Model file for the job. Use its own axes, mm. A direction names the side the tool comes from. Round coordinates to 2 decimals unless told otherwise and drop trailing zeros. Order: outer loops, then holes, each group sorted by start corner. A loop starts at its lowest first (then second) coordinate and runs counter-clockwise, first axis right, second up. Notation, with made-up numbers: (-8, 12) - (43, 12) arc R23 ccw to (43, 26) - close; hole circle Ø8 at (80, 82). An arc over 180 degrees is marked (long way). Write item = value, one per line.
Autodesk Inventor part; units mm, degrees
ref_plane "YZ Plane" through (0, 0, 0) normal (1, 0, 0) x (0, 1, 0)
ref_plane "XZ Plane" through (0, 0, 0) normal (0, 1, 0) x (-1, 0, 0)
ref_plane "XY Plane" through (0, 0, 0) normal (0, 0, 1) x (1, 0, 0)
sketch "草圖1" plane through (0, 0, 0) normal (0, 1, 0) x (-1, 0, 0)
  line L0 (0, 0) -> (-8, 0)
  line L1 (-8, 0) -> (-8, -30)
  line L2 (0, 0) -> (0, -30)
  arc A0 (-42, -30) -> (-8, -30) centre (-25, -30) ccw
  arc A1 (-50, -30) -> (0, -30) centre (-25, -30) ccw
  line L3 (6.1696, -30) -> (-69.0697, -30) construction
  line L4 (-25, -30) -> (-25, -20.8656)
  line L5 (-42, 0) -> (-42, -30)
  line L6 (-50, 0) -> (-50, -30)
  line L7 (-42, 0) -> (-50, 0)
  dimension "d8" = 30
  dimension "d9" = 8
  dimension "d10" = 25
  dimension "d11" = 17
extrude "擠出1" add sketch "草圖1" along normal blind 10
sketch "草圖2" plane through (0, 10, 0) normal (0, 1, 0) x (1, 0, 0)
  line L0 (0, 30) -> (0, 0)
  line L1 (0, 0) -> (0, 20)
  line L2 (0, 20) -> (8, 20)
  line L3 (8, 0) -> (8, 30)
  line L4 (8, 20) -> (8, 0)
  line L5 (8, 0) -> (0, 0)
  arc A0 (42, 30) -> (8, 30) centre (25, 30) ccw
  line L6 (25, 30) -> (25, 60.7006)
  line L7 (50, 20) -> (50, 0)
  line L8 (50, 0) -> (50, 20)
  line L9 (50, 20) -> (42, 20)
  line L10 (42, 0) -> (42, 20)
  line L11 (42, 20) -> (42, 0)
  line L12 (42, 0) -> (50, 0)
  point P0 (50, 30)
  dimension "d14" = 20
extrude "擠出2" add sketch "草圖2" along normal blind 30
sketch "草圖3" plane through (0, 40, 0) normal (0, 1, 0) x (1, 0, 0)
  line L0 (0, 20) -> (8, 20)
  line L1 (8, 20) -> (8, 30)
  arc A0 (42, 30) -> (8, 30) centre (25, 30) ccw
  line L2 (42, 30) -> (42, 20)
  line L3 (42, 20) -> (50, 20)
  line L4 (50, 20) -> (50, 30)
  arc A1 (50, 30) -> (0, 30) centre (25, 30) ccw
  line L5 (0, 30) -> (0, 20)
  line L6 (0, 0) -> (8, 0)
  line L7 (8, 0) -> (8, 20)
  line L8 (8, 20) -> (0, 20)
  line L9 (0, 20) -> (0, 0)
  line L10 (50, 0) -> (50, 20)
  line L11 (50, 20) -> (42, 20)
  line L12 (42, 20) -> (42, 0)
  line L13 (42, 0) -> (50, 0)
extrude "擠出3" add sketch "草圖3" along normal blind 10
properties part number "410571040示範三"
1) Flat gauge pins, fed straight in: pin 1 Ø4 at (x, y) = (46.5, 17.5) entering from -Z; pin 2 Ø3 at (x, y) = (37, 42) entering from +Z. Where does each tip first touch, or does it go through?
Conclusion:
pin_1 = -20
pin_2 = -40.33
2) Cut at B-B (x = 25). Write the cut outline in (y, z), and give its area (3 significant figures).
Conclusion:
outline = (0, -55) - (10, -55) - (10, -47) - (0, -47) - close; (40, -55) - (50, -55) - (50, -47) - (40, -47) - close
area = 160 mm^2
3) Cut at D-D (z = -37). Write the cut outline in (x, y).
Conclusion:
outline = (1, 0) - (9.51, 0) - (9.51, 10) - (1, 10) - close; (1, 40) - (9.51, 40) - (9.51, 50) - (1, 50) - close; (40.49, 0) - (49, 0) - (49, 10) - (40.49, 10) - close; (40.49, 40) - (49, 40) - (49, 50) - (40.49, 50) - close
4) Wall check: line 1 along X through (y, z) = (3.5, -10); line 2 along Y through (x, z) = (7, -27.5); line 3 along Z through (x, y) = (44, 27). Give the ranges that are in metal, low to high.
Conclusion:
line_1 = 0 to 8, 42 to 50
line_2 = 0 to 10, 40 to 50
line_3 = -20 to 0
5) 3-axis set-ups, long thin cutter, end or side, ignore diameter. For faces 5 (the face through (42, 25, -11)), 6 (the face through (25, 10, -49)), 7 (the face through (50, 25, -11)): which of +Z, -Z, +X, -X, +Y, -Y reach the whole face in a straight line?
Conclusion:
face_5 = +Z, +Y, -Y
face_6 = -Z, +X, -X
face_7 = +Z, -Z, +X, +Y, -Y
6) Cut at C-C (y = 3). Write the cut outline in (x, z).
Conclusion:
outline = (0, -30) arc R25 ccw to (50, -30) - (50, 0) - (42, 0) - (42, -30) arc R17 cw to (8, -30) - (8, 0) - (0, 0) - close
7) Mould opens along Y. For faces 1 (the face through (25, 45, -47)), 2 (the face through (4, 25, -20)), 3 (the face through (8, 50, -34)), 4 (the face through (46, 25, -20)) say: +Y half, -Y half, draft (parallel to the pull), parting line (faces both ways), or undercut.
Conclusion:
face_1 = draft
face_2 = undercut
face_3 = +Y half
face_4 = undercut
8) Cut at A-A (z = -23). Write the cut outline in (x, y), and give its area (3 significant figures).
Conclusion:
outline = (0, 0) - (8, 0) - (8, 10) - (0, 10) - close; (0, 40) - (8, 40) - (8, 50) - (0, 50) - close; (42, 0) - (50, 0) - (50, 10) - (42, 10) - close; (42, 40) - (50, 40) - (50, 50) - (42, 50) - close
area = 320 mm^2
